Geometry: final body of the model. Coordinates: model frame, mm. Face numbers are marked on the shaded views. A direction names the side the tool comes from. Round coordinates to 2 decimals unless told otherwise and drop trailing zeros. Write each loop counter-clockwise with the first axis right and the second up, starting at its lowest first coordinate (ties: lowest second). Pieces come first, ordered by that corner, then holes. Notation, with made-up numbers: (11.25, 53.25) -> (33.25, 53.25) arc R13 ccw to (33.25, 70.25) -> close; hole circle Ø8 at (56.5, 50). An arc over 180 degrees is marked (long way). Use one line per item in the form item = value. Start each with the question number.
1. Reachability of the marked faces 3, 4 and 5 from +Z, -Z, +X, -X, +Y, -Y: full face, straight path, thin tool, end or side. Return the list, or none.
2. Cut plane A-A, the plane z = 0. Return the cut outline in (x, y).
3. Cut plane C-C, the plane z = -7.5. Return the cut outline in (x, y), plus the area to 3 significant figures.
4. Cut plane B-B, the plane x = -30. Return the cut outline in (y, z).
5. Draft query along X for the marked faces 1 and 2. Return one class per face: pulls with the +X half, pulls with the -X half, needs draft (parallel to the pull), parting line crosses it, or undercut.
6. Line query: L1, parallel to X at y = 2.35, z = 0; L2, parallel to Z at x = -30, y = 3.2; L3, parallel to X at y = 0.8, z = -1.25. Output: solid intervals per line, ascending.
7. Pin query (flat end, axial travel): pin 1 Ø2.5 at (x, y) = (-7.5, 1.5) entering from -Z; pin 2 Ø1 at (y, z) = (3, -5) entering from +X; pin 3 Ø1 at (x, y) = (4.5, 1) entering from +Z. Return the tip coordinate at first contact, or that it passes through.
8. Cut plane D-D, the plane y = 4.15. Return the cut outline in (x, z).
```python
from build123d import *

# Parameters (mm, degrees)
SKIZZE1_R                       = 2
AUFSATZ_LINEAR_AUSTRAGEN1_DEPTH = 5


with BuildPart() as part:
    # Skizze1 → Aufsatz-Linear austragen1 (new body)
    with BuildSketch(Plane(origin=(0, 0, 0), x_dir=(1, 0, 0), z_dir=(0, 1, 0))):
        with BuildLine():
            Line((22.400657923, 6.5), (0, 6.5))
            Line((0, 6.5), (0, -6.5))
            Line((0, -6.5), (22.400657923, -6.5))
            ThreePointArc((22.400657923, -6.5), (40, 0), (22.400657923, 6.5))
        make_face()
        with Locations(Location((30, 0, 0), (0, 0, 270))):
            Circle(SKIZZE1_R, mode=Mode.SUBTRACT)
    aufsatz_linear_austragen1 = extrude(amount=AUFSATZ_LINEAR_AUSTRAGEN1_DEPTH)

    # Spiegeln1: Aufsatz-Linear austragen1 across plane
    add(aufsatz_linear_austragen1.mirror(Plane(origin=(0, 0, 0), x_dir=(0, 0, 1), z_dir=(1, 0, 0))))


solid = part.part
```
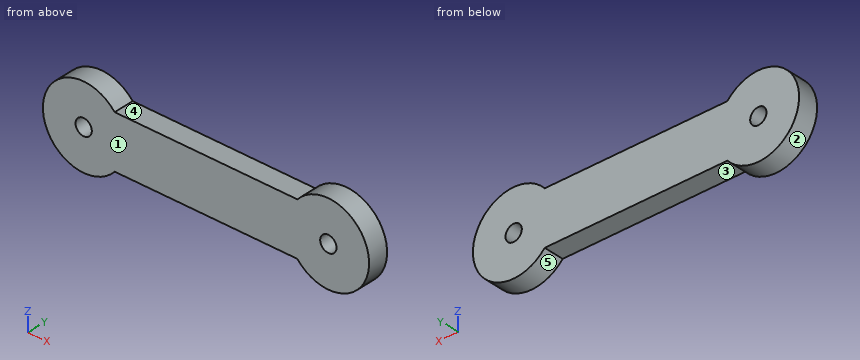
Outcome:
q1.face_3 = -Z, +Y, -Y
q1.face_4 = +Z, +Y, -Y
q1.face_5 = +Y, -Y
q2.outline = (-40, 0) -> (-32, 0) -> (-32, 5) -> (-40, 5) -> close; (-28, 0) -> (28, 0) -> (28, 5) -> (-28, 5) -> close; (32, 0) -> (40, 0) -> (40, 5) -> (32, 5) -> close
q3.outline = (-36.61, 0) -> (-23.39, 0) -> (-23.39, 5) -> (-36.61, 5) -> close; (23.39, 0) -> (36.61, 0) -> (36.61, 5) -> (23.39, 5) -> close
q3.area = 132 mm^2
q4.outline = (0, -10) -> (5, -10) -> (5, -2) -> (0, -2) -> close; (0, 2) -> (5, 2) -> (5, 10) -> (0, 10) -> close
q5.face_1 = needs draft
q5.face_2 = undercut
q6.L1 = -40 to -32, -28 to 28, 32 to 40
q6.L2 = -10 to -2, 2 to 10
q6.L3 = -39.92 to -31.56, -28.44 to 28.44, 31.56 to 39.92
q7.pin_1 = -6.5
q7.pin_2 = 38.93
q7.pin_3 = 6.5
q8.outline = (-22.4, -6.5) -> (22.4, -6.5) arc R10 ccw (long way) to (22.4, 6.5) -> (-22.4, 6.5) arc R10 ccw (long way) to start; hole circle Ø4 at (-30, 0); hole circle Ø4 at (30, 0)
